from build123d import *

# Parameters (mm, degrees)
BOSS_EXTRUDE1_DEPTH = 5
SKETCH2_R           = 6.5
BOSS_EXTRUDE2_DEPTH = 0.3
SKETCH3_R           = 4
BOSS_EXTRUDE3_DEPTH = 50


with BuildPart() as part:
    # Sketch1 → Boss-Extrude1 (new body)
    with BuildSketch(Plane(origin=(0, 0, 0), x_dir=(0, 0, -1), z_dir=(1, 0, 0))):
        Polygon((-7.505553499, 0), (-3.75277675, -6.5), (3.75277675, -6.5), (7.505553499, 0), (3.75277675, 6.5), (-3.75277675, 6.5), align=None)
    extrude(amount=-BOSS_EXTRUDE1_DEPTH)

    # Sketch2 → Boss-Extrude2 (add)
    with BuildSketch(Plane(origin=(0, 0, 0), x_dir=(0, 0, -1), z_dir=(1, 0, 0))):
        with Locations(Location((0, 0, 0), (0, 0, 150))):
            Circle(SKETCH2_R)
    extrude(amount=BOSS_EXTRUDE2_DEPTH)

    # Sketch3 → Boss-Extrude3 (add)
    with BuildSketch(Plane(origin=(0.3, 0, 0), x_dir=(0, 0, -1), z_dir=(1, 0, 0))):
        Circle(SKETCH3_R)
    extrude(amount=BOSS_EXTRUDE3_DEPTH)


solid = part.part
Work out the finished part from the listing and answer in its coordinate system (mm). A direction names the side the tool comes from. Round coordinates to 2 decimals unless told otherwise and drop trailing zeros. Loops run counter-clockwise (first coordinate to the right, second up) from the corner with the lowest first, then second, coordinate; pieces in that order, holes last. Notation, with made-up numbers: (60.5, 21.25) - (97.5, 21.25) arc R15 cw to (97.5, 43.25) - close; hole circle Ø5 at (84, -15.5). An arc over 180 degrees is marked (long way). Use one line per item in the form item = value. Start each with the question number.
(1) Which of the six approach directions +Z, -Z, +X, -X, +Y, -Y give full straight-line access (tool end or side, diameter ignored) to faces 1 (the face through (0, -6, -3)), 2 (the face through (0, 0, -7)), 3 (the face through (0, 6, -3))?
(2) Flat-ended cylindrical pins translate along their axes: P1, Ø1.5, axis at x = 36.5, z = -3, coming from the +Y side; P2, Ø1.5, axis at y = -1, z = -7, coming from the +X side; P3, Ø4, axis at x = 5, y = 4.5, coming from the -Z side. Find the tip coordinate at first contact, or state that the pin passes through.
(3) Consider line 1 (X direction, y = -4.5, z = 1.5); line 2 (Z direction, x = 13, y = -0.25). Determine where each line is inside the solid, lowest interval first.
(4) Find section D-D on y = 0.75. Determine the outline of the cut face in (x, z).
(5) Find section A-A on z = 3. Determine the outline of the cut face in (x, y).
(6) Find section B-B on y = 5.25. Determine the outline of the cut face in (x, z).
(7) Find section C-C on x = 22. Determine the outline of the cut face in (y, z), and give its area (3 significant figures).
Answer list:
q1.face_1 = -Z, +X, -Y
q1.face_2 = -Z, +X
q1.face_3 = -Z, +X, +Y
q2.P1 = 3.31
q2.P2 = 0.3
q2.P3 = -3.12
q3.line_1 = -5 to 0.3
q3.line_2 = -3.99 to 3.99
q4.outline = (-5, -7.07) - (0, -7.07) - (0, -6.46) - (0.3, -6.46) - (0.3, -3.93) - (50.3, -3.93) - (50.3, 3.93) - (0.3, 3.93) - (0.3, 6.46) - (0, 6.46) - (0, 7.07) - (-5, 7.07) - close
q5.outline = (-5, -6.5) - (0, -6.5) - (0, -5.77) - (0.3, -5.77) - (0.3, -2.65) - (50.3, -2.65) - (50.3, 2.65) - (0.3, 2.65) - (0.3, 5.77) - (0, 5.77) - (0, 6.5) - (-5, 6.5) - close
q6.outline = (-5, -4.47) - (0, -4.47) - (0, -3.83) - (0.3, -3.83) - (0.3, 3.83) - (0, 3.83) - (0, 4.47) - (-5, 4.47) - close
q7.outline = circle Ø8 at (0, 0)
q7.area = 50.3 mm^2
